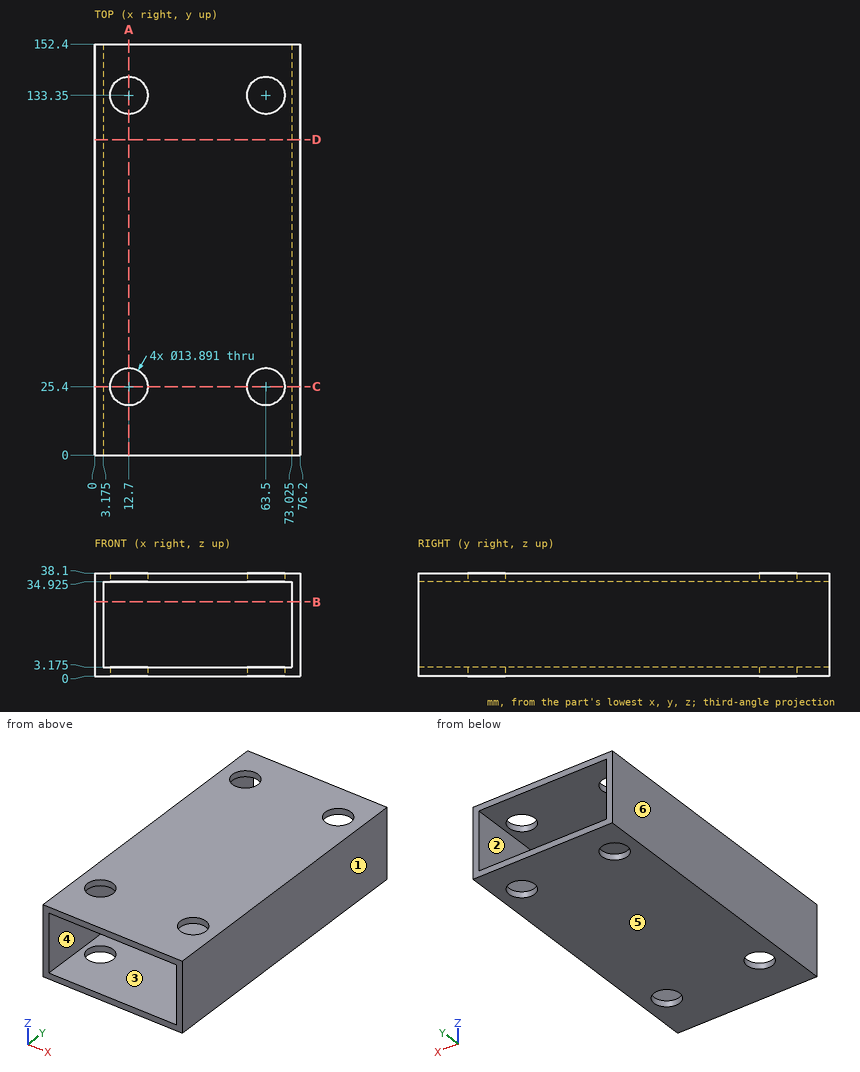
Verification items for this drawing (mm, ordinates from the low corner). A direction names the side the tool comes from. Give positions to 0.01 mm unless a question says otherwise; leave off trailing zeros. Loops run counter-clockwise (first coordinate to the right, second up) from the corner with the lowest first, then second, coordinate; pieces in that order, holes last. Notation, with made-up numbers: M 13,67.25 L 49,67.25 A7 ccw 49,79.25 Z; hole C 8.5,50 d11. An arc over 180 degrees is marked long. Write item = value, one per line. Start each with the question number.
1. Draft check along Z on the marked faces 3, 4, 5 and 6. Enter one of: +Z half, -Z half, draft (parallel to the pull), parting line (faces both ways), or undercut.
2. Thickness scan on probe 1 along X at (y, z) = (133, 35); probe 2 along Y at (x, z) = (12.7, 2.3); probe 3 along Z at (x, y) = (38, 91) (1 decimal). Record the ranges inside material, lowest first.
3. Section check D-D, the plane y = 117. Enter the section's corners in (x, z) (1 decimal).
4. Section check A-A, the plane x = 12.7. Enter the section's corners in (y, z) (1 decimal).
5. Section check C-C, the plane y = 25.4. Enter the section's corners in (x, z) (1 decimal), plus the area to 3 significant figures.
6. Tool access check on the marked faces 1 and 2. Record the directions out of +Z, -Z, +X, -X, +Y, -Y that give a thin tool (end or side, any length) a straight path to the whole face; none if there is none.
7. Section check B-B, the plane z = 27.5. Enter the section's corners in (x, y) (1 decimal).
8. Go/stop test with a flat-tipped pin: P1, Ø12.5, axis at x = 12.7, y = 25.4, coming from the -Z side. Record where the tip stops, or that it passes through.
Values follow:
q1.face_3 = undercut
q1.face_4 = undercut
q1.face_5 = -Z half
q1.face_6 = draft
q2.probe_1 = 0 to 5.76, 19.64 to 56.56, 70.44 to 76.2
q2.probe_2 = 0 to 18.45, 32.35 to 126.4, 140.3 to 152.4
q2.probe_3 = 0 to 3.2, 34.9 to 38.1
q3.outline = M 0,0 L 76.2,0 L 76.2,38.1 L 0,38.1 Z; hole M 3.2,3.2 L 73,3.2 L 73,34.9 L 3.2,34.9 Z
q4.outline = M 0,0 L 18.5,0 L 18.5,3.2 L 0,3.2 Z; M 0,34.9 L 18.5,34.9 L 18.5,38.1 L 0,38.1 Z; M 32.3,0 L 126.4,0 L 126.4,3.2 L 32.3,3.2 Z; M 32.3,34.9 L 126.4,34.9 L 126.4,38.1 L 32.3,38.1 Z; M 140.3,0 L 152.4,0 L 152.4,3.2 L 140.3,3.2 Z; M 140.3,34.9 L 152.4,34.9 L 152.4,38.1 L 140.3,38.1 Z
q5.outline = M 0,0 L 5.8,0 L 5.8,3.2 L 3.2,3.2 L 3.2,34.9 L 5.8,34.9 L 5.8,38.1 L 0,38.1 Z; M 19.6,0 L 56.6,0 L 56.6,3.2 L 19.6,3.2 Z; M 19.6,34.9 L 56.6,34.9 L 56.6,38.1 L 19.6,38.1 Z; M 70.4,0 L 76.2,0 L 76.2,38.1 L 70.4,38.1 L 70.4,34.9 L 73,34.9 L 73,3.2 L 70.4,3.2 Z
q5.area = 509 mm^2
q6.face_1 = +Z, -Z, +X, +Y, -Y
q6.face_2 = +Y, -Y
q7.outline = M 0,0 L 3.2,0 L 3.2,152.4 L 0,152.4 Z; M 73,0 L 76.2,0 L 76.2,152.4 L 73,152.4 Z
q8.P1 = through
